```python
from build123d import *

# Parameters (mm, degrees)
CYLINDER1020_R     = 2.7
CYLINDER1020_DEPTH = 10
CYLINDER1018_R     = 1.7
CYLINDER1018_DEPTH = 10


with BuildPart() as cylinder1015:
    # Cylinder1020 → Cylinder1020 (new body)
    with BuildSketch(Plane.XY.offset(10)):
        Circle(CYLINDER1020_R)
    extrude(amount=CYLINDER1020_DEPTH)


with BuildPart() as m3bolthead:
    # Cylinder1018 → Cylinder1018 (new body)
    with BuildSketch(Plane.XY):
        Circle(CYLINDER1018_R)
    extrude(amount=CYLINDER1018_DEPTH)

    # Fusion024: union Cylinder1015
    add(cylinder1015.part)


solid = m3bolthead.part
```
Work out the finished part from the listing and answer in its coordinate system (mm). A direction names the side the tool comes from. Give positions to 0.01 mm unless a question says otherwise; leave off trailing zeros. Write each loop counter-clockwise with the first axis right and the second up, starting at its lowest first coordinate (ties: lowest second). Pieces come first, ordered by that corner, then holes. Notation, with made-up numbers: (-37, -21) -> (21, -21) arc R34 cw to (21, 15) -> close; hole circle Ø6 at (-24, -24.5). An arc over 180 degrees is marked (long way). Write item = value, one per line.
Q1. Section D-D on z = 11.25 is taken. Determine the outline of the cut face in (x, y), and give its area (3 significant figures).
Computed values:
outline = circle Ø5.4 at (0, 0)
area = 22.9 mm^2
Q2. A tool of negligible diameter and unlimited length cuts with its end or side. For faces 1 (the flat face through (0, -2, 10)), 2 (the flat face through (0, 0, 20)), from which of +Z, -Z, +X, -X, +Y, -Y can it reach the whole face along a straight path? Write none if from no direction.
Computed values:
face_1 = -Z
face_2 = +Z, +X, -X, +Y, -Y
Q3. Consider line 1 along X through (y, z) = (-2.1, 10.25); line 2 along Z through (x, y) = (1.25, -1.4). Determine where each line is inside the solid, lowest interval first.
Computed values:
line_1 = -1.7 to 1.7
line_2 = 10 to 20
Q4. Section C-C on z = 4.5 is taken. Determine the outline of the cut face in (x, y).
Computed values:
outline = circle Ø3.4 at (0, 0)
Q5. Section A-A on x = 0 is taken. Determine the outline of the cut face in (y, z), and give its area (3 significant figures).
Computed values:
outline = (-2.7, 10) -> (-1.7, 10) -> (-1.7, 0) -> (1.7, 0) -> (1.7, 10) -> (2.7, 10) -> (2.7, 20) -> (-2.7, 20) -> close
area = 88.0 mm^2
Q6. Flat-ended cylindrical pins translate along their axes: pin 1 Ø1.5 at (y, z) = (1.5, 11.5) entering from +X; pin 2 Ø3 at (y, z) = (-1, 6) entering from -X. Find the tip coordinate at first contact, or state that the pin passes through.
Computed values:
pin_1 = 2.59
pin_2 = -1.7
